```python
from build123d import *

# Parameters (mm, degrees)
F0_R     = 190.5
F1_DEPTH = 152.4
F1_TAPER = -10
F2_R     = 31.115
F3_DEPTH = 88.9
F4_R     = 209.1526888915
F5_DEPTH = 76.2
F5_TAPER = 10


with BuildPart() as f1:
    # F0 (on Top) → F1 (new body)
    with BuildSketch(Plane.XY):
        Circle(F0_R)
    extrude(amount=F1_DEPTH, taper=F1_TAPER)

    # F2 (on face) → F3 (cut)
    with BuildSketch(Plane.XY.offset(152.4)):
        Circle(F2_R)
    extrude(amount=-F3_DEPTH, mode=Mode.SUBTRACT)

    # F4 (on face) → F5 (cut)
    with BuildSketch(Plane.XY.offset(152.4)):
        Circle(F4_R)
    extrude(amount=-F5_DEPTH, taper=F5_TAPER, mode=Mode.SUBTRACT)


solid = f1.part
```
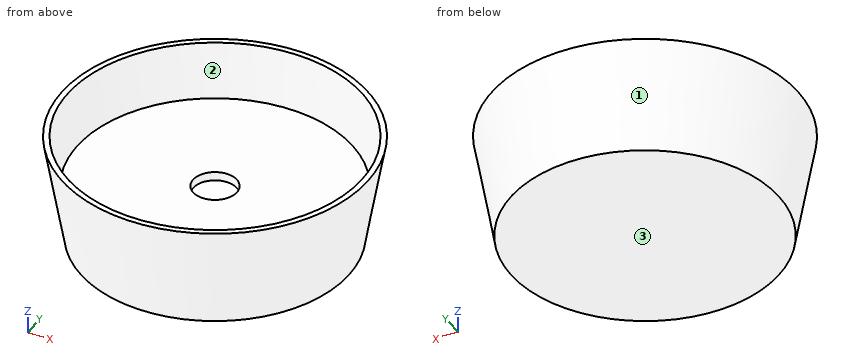
Can you work these out from the model? Positions are in its coordinate system, mm. Face numbers are marked on the shaded views. Coordinates: 2 decimals unless noted, no trailing zeros. Loops run counter-clockwise (first coordinate to the right, second up) from the corner with the lowest first, then second, coordinate; pieces in that order, holes last.
Item 1: I'm going to push flat-ended pins straight in: pin 1 (1 mm diameter, centred on x = 108.5, z = 87.5, fed in from -Y); pin 2 (12 mm diameter, centred on y = -13, z = 20.5, fed in from +X); pin 3 (10 mm diameter, centred on x = 81.5, y = -49, fed in from +Z). Where does each tip first touch, or does it pass through?
Answers below:
pin 1: stops at y = -175.35
pin 2: stops at x = 194.8
pin 3: stops at z = 76.2
Item 2: Suppose I cut it at A-A (x = 0). Please give me the cut outline in (y, z) (3 decimals).
Answers below:
outline: (-217.372, 152.4) - (-190.5, 0) - (190.5, 0) - (217.372, 152.4) - (209.153, 152.4) - (195.717, 76.2) - (31.115, 76.2) - (31.115, 63.5) - (-31.115, 63.5) - (-31.115, 76.2) - (-195.717, 76.2) - (-209.153, 152.4) - close
Item 3: Suppose I cut it at B-B (z = 129). Please give me the cut outline in (x, y).
Answers below:
outline: circle Ø426.49 at (0, 0); hole circle Ø410.05 at (0, 0)
Item 4: Please list where these lines run through material, in increasing order: L1, parallel to Z at x = 176, y = 49; L2, parallel to Y at x = 126.5, z = 119.5; L3, parallel to X at y = 183.5, z = 120.
Answers below:
L1: z = 0 to 76.2
L2: y = -169.59 to -159.22, 159.22 to 169.59
L3: x = -105.49 to -87.84, 87.84 to 105.49
Item 5: If we mould it in two halves opening along Y, with no side actions, what happens to the marked faces 1, 2 and 3? For each: released by +Y, released by -Y, zero draft, split by the parting line, or undercut.
Answers below:
face 1: split by the parting line
face 2: undercut
face 3: zero draft
